Geometry: final body of the model. Coordinates: model frame, mm. A direction names the side the tool comes from. Give positions to 0.01 mm unless a question says otherwise; leave off trailing zeros. Write each loop counter-clockwise with the first axis right and the second up, starting at its lowest first coordinate (ties: lowest second). Pieces come first, ordered by that corner, then holes. Notation, with made-up numbers: (43, 24) -> (52, 24) arc R14 ccw to (52, 33) -> close; hole circle Ø3 at (47, -23). An arc over 180 degrees is marked (long way). Answer as a JSON object with one key per item and string values. Group by question number.
(1) Section query B-B on x = -12. Output: boundary loops of the cut face in (y, z), plus the area to 3 significant figures.
(2) Material intervals for probe 1 along X at (y, z) = (2.75, -0.75); probe 2 along Z at (x, y) = (-14, 1.25); probe 3 along Z at (x, y) = (0, 4.55), sorted ascending.
(3) Draft query along X for faces 1 (the face through (-3.866, 2.958, -2.471)), 2 (the face through (16, 1, 0)), 3 (the face through (3.907, 2.958, -2.486)), 4 (the face through (-11, 2, 0)). Return one class per face: +X half, -X half, draft (parallel to the pull), parting line (faces both ways), or undercut.
(4) Contact query for flat-ended pins moving along their axis: pin 1 Ø4 at (x, z) = (-5.5, -1) entering from +Y; pin 2 Ø1 at (x, y) = (12.5, 1.5) entering from -Z; pin 3 Ø0.6 at (x, y) = (-11.5, 1.5) entering from +Z; pin 4 Ø1 at (y, z) = (3.5, 2) entering from +X. Output: stop coordinate, or through.
(5) Set-up query: faces 5 (the face through (11, 1, -1.9)), 6 (the face through (11, 1, 1.9)), 7 (the face through (-11, 1, 1.9)). Return all of +Z, -Z, +X, -X, +Y, -Y with unobstructed straight access to the full face (end or side cutting, diameter ignored); none if empty.
(6) Section query C-C on y = 3.45. Output: boundary loops of the cut face in (x, z).
(7) Section query D-D on x = 0. Output: boundary loops of the cut face in (y, z), plus the area to 3 significant figures.
(8) Section query A-A on z = 1.5. Output: boundary loops of the cut face in (x, y), plus the area to 3 significant figures.
from build123d import *

# Parameters (mm, degrees)
BOSS_EXTRUDE1_DEPTH = 6
SKETCH2_W           = 11.5
SKETCH2_H           = 3.8
SKETCH2_H_2         = 1.9
BOSS_EXTRUDE2_DEPTH = 2


with BuildPart() as part:
    # Sketch1 → Boss-Extrude1 (new body)
    with BuildSketch(Plane(origin=(0, 0, 0), x_dir=(1, 0, 0), z_dir=(0, 1, 0))):
        with BuildLine():
            Line((5.5, 0), (3.5, 0))
            ThreePointArc((3.5, 0), (-0.607768622, -3.446827136), (-3.288924173, 1.197070502))
            ThreePointArc((-3.288924173, 1.197070502), (-3.88659665, 2.478783266), (-5.168309414, 1.881110788))
            ThreePointArc((-5.168309414, 1.881110788), (-0.955064977, -5.416442642), (5.5, 0))
        make_face()
        with BuildLine():
            ThreePointArc((3.288924173, 1.197070502), (3.446827136, 0.607768622), (3.5, 0))
            Line((3.5, 0), (5.5, 0))
            ThreePointArc((5.5, 0), (5.416442642, 0.955064977), (5.168309414, 1.881110788))
            Line((5.168309414, 1.881110788), (4.228616794, 1.539090645))
            Line((4.228616794, 1.539090645), (3.288924173, 1.197070502))
        make_face()
        with BuildLine():
            ThreePointArc((5.168309414, 1.881110788), (3.88659665, 2.478783266), (3.288924173, 1.197070502))
            Line((3.288924173, 1.197070502), (4.228616794, 1.539090645))
            Line((4.228616794, 1.539090645), (5.168309414, 1.881110788))
        make_face()
    extrude(amount=BOSS_EXTRUDE1_DEPTH)

    # Sketch2 → Boss-Extrude2 (add)
    with BuildSketch(Plane(origin=(0, 0, 0), x_dir=(1, 0, 0), z_dir=(0, 1, 0))):
        with Locations((-10.25, 0)):
            Rectangle(SKETCH2_W, SKETCH2_H)
        with Locations((10.25, -0.95)):
            Rectangle(SKETCH2_W, SKETCH2_H_2)
        with Locations((10.25, 0.95)):
            Rectangle(SKETCH2_W, SKETCH2_H_2)
    extrude(amount=BOSS_EXTRUDE2_DEPTH)


solid = part.part
Answer list:
{
 "1": {"outline": "(0, -1.9) -> (2, -1.9) -> (2, 1.9) -> (0, 1.9) -> close", "area": "7.60 mm2"},
 "2": {"probe 1": "-5.45 to -3.42, 3.42 to 5.45", "probe 2": "-1.9 to 1.9", "probe 3": "3.5 to 5.5"},
 "3": {"face 1": "undercut", "face 2": "+X half", "face 3": "undercut", "face 4": "draft"},
 "4": {"pin 1": "y = 6", "pin 2": "z = -1.9", "pin 3": "z = 1.9", "pin 4": "x = 5.29"},
 "5": {"face 5": "-Z, +X, +Y, -Y", "face 6": "+Z, +X, +Y, -Y", "face 7": "+Z, -X, +Y, -Y"},
 "6": {"outline": "(-5.17, -1.88) arc R1 ccw to (-3.29, -1.2) arc R3.5 cw (long way) to (3.29, -1.2) arc R1 ccw to (5.17, -1.88) arc R5.5 ccw (long way) to start"},
 "7": {"outline": "(0, 3.5) -> (6, 3.5) -> (6, 5.5) -> (0, 5.5) -> close", "area": "12.0 mm2"},
 "8": {"outline": "(-16, 0) -> (-3.16, 0) -> (-3.16, 6) -> (-5.29, 6) -> (-5.29, 2) -> (-16, 2) -> close; (3.16, 0) -> (16, 0) -> (16, 2) -> (5.29, 2) -> (5.29, 6) -> (3.16, 6) -> close", "area": "68.4 mm2"}
}
